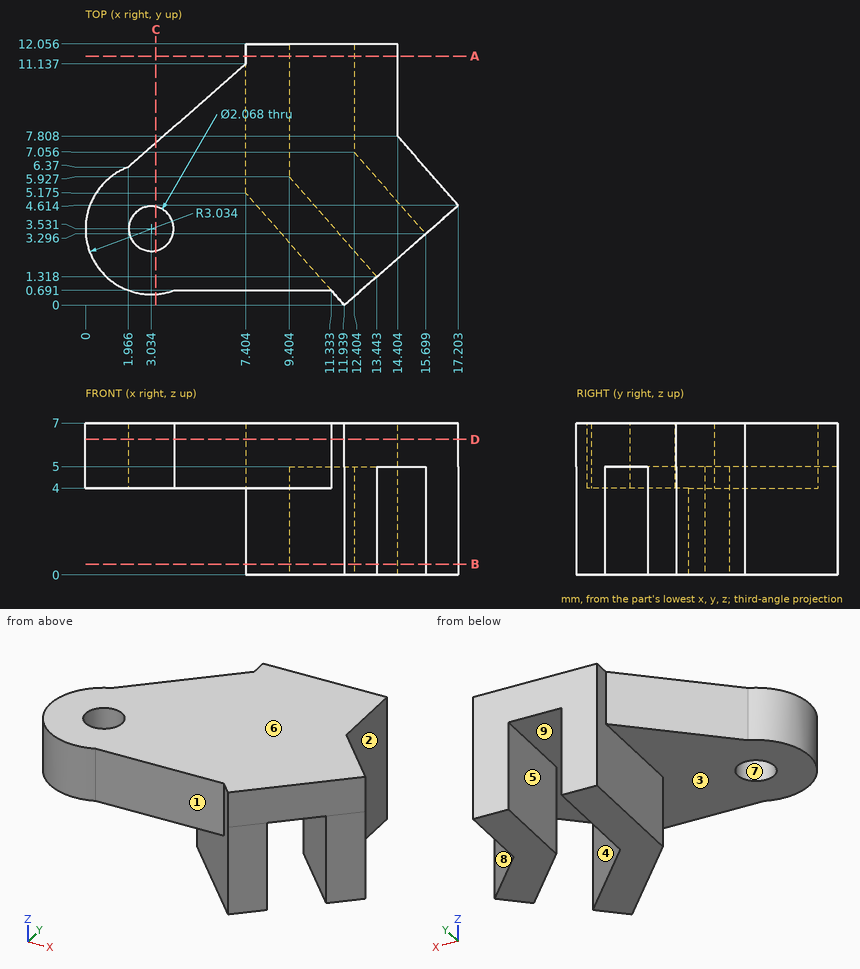
Geometry: see drawing. Coordinates: mm, zero at the bounding-box minimum. A direction names the side the tool comes from. Round coordinates to 2 decimals unless told otherwise and drop trailing zeros. Write each loop counter-clockwise with the first axis right and the second up, starting at its lowest first coordinate (ties: lowest second). Pieces come first, ordered by that corner, then holes. Notation, with made-up numbers: M -8.75,-37.5 L 50.25,-37.5 A14 cw 50.25,-33.5 Z; hole C 58.5,6.5 d5. An arc over 180 degrees is marked long. Answer in a Markdown table with one row per item. Add a question column.
(1) Ray query, L1, parallel to Z at x = 5.75, y = 4.25; L2, parallel to X at y = 10.25, z = 1.5; L3, parallel to X at y = 6.25, z = 0.5 (1 decimal). Return the intervals inside material, ascending.
(2) Cut plane A-A, the plane y = 11.5. Return the cut outline in (x, z), then the cut area to 3 significant figures.
(3) Cut plane D-D, the plane z = 6.25. Return the cut outline in (x, y) (1 decimal), then the cut area to 3 significant figures.
(4) Cut plane B-B, the plane z = 0.5. Return the cut outline in (x, y) (1 decimal).
(5) Cut plane C-C, the plane x = 3.25. Return the cut outline in (y, z) (1 decimal), then the cut area to 3 significant figures.
(6) Contact query for flat-ended pins moving along their axis: pin 1 (3.5 mm diameter, centred on x = 3.03, y = 3.53, fed in from -Z); pin 2 (2.5 mm diameter, centred on x = 6, z = 5.5, fed in from -Y); pin 3 (3.5 mm diameter, centred on y = 9.5, z = 3, fed in from +X) (1 decimal); pin 4 (3 mm diameter, centred on x = 7, y = 5.5, fed in from -Z). Output: stop coordinate, or through.
(7) Draft query along X for the marked faces 6, 7, 8 and 9. Return one class per face: pulls with the +X half, pulls with the -X half, needs draft (parallel to the pull), parting line crosses it, or undercut.
(8) Reachability of the marked faces 1, 2, 3, 4 and 5 from +Z, -Z, +X, -X, +Y, -Y: full face, straight path, thin tool, end or side. Return the list, or none.
Established:
| question | item | result |
|---|---|---|
| 1 | L1 | 4 to 7 |
| 1 | L2 | 7.4 to 9.4, 12.4 to 14.4 |
| 1 | L3 | 7.4 to 9.4, 13.1 to 15.8 |
| 2 | outline | M 7.4,0 L 9.4,0 L 9.4,5 L 12.4,5 L 12.4,0 L 14.4,0 L 14.4,7 L 7.4,7 Z |
| 2 | area | 34.0 mm² |
| 3 | outline | M 2,6.4 A3 ccw 4.1,0.7 L 11.3,0.7 L 11.9,0 L 17.2,4.6 L 14.4,7.8 L 14.4,12.1 L 7.4,12.1 L 7.4,11.1 Z; hole C 3,3.5 d2.1 |
| 3 | area | 136 mm² |
| 4 | outline | M 7.4,5.2 L 11.9,0 L 13.4,1.3 L 9.4,5.9 L 9.4,12.1 L 7.4,12.1 Z; M 12.4,7.1 L 15.7,3.3 L 17.2,4.6 L 14.4,7.8 L 14.4,12.1 L 12.4,12.1 Z |
| 5 | outline | M 0.5,4 L 2.5,4 L 2.5,7 L 0.5,7 Z; M 4.5,4 L 7.5,4 L 7.5,7 L 4.5,7 Z |
| 5 | area | 14.9 mm² |
| 6 | pin 1 | z = 4 |
| 6 | pin 2 | y = 0.69 |
| 6 | pin 3 | x = 14.5 |
| 6 | pin 4 | z = 0 |
| 7 | face 6 | needs draft |
| 7 | face 7 | undercut |
| 7 | face 8 | pulls with the +X half |
| 7 | face 9 | undercut |
| 8 | face 1 | +Z, -Z, -Y |
| 8 | face 2 | +Z, -Z, +X, +Y |
| 8 | face 3 | -Z, -X, -Y |
| 8 | face 4 | -Z |
| 8 | face 5 | -Z, +Y |
